Verification items for the finished model (mm, model axes). Face numbers are marked on the shaded views. A direction names the side the tool comes from. Round coordinates to 2 decimals unless told otherwise and drop trailing zeros. Order: outer loops, then holes, each group sorted by start corner. A loop starts at its lowest first (then second) coordinate and runs counter-clockwise, first axis right, second up. Notation, with made-up numbers: M 45.5,61 L 50.5,61 A25 ccw 50.5,81 Z; hole C 31.5,72 d8. An arc over 180 degrees is marked long. Use CSV: the item, a comma, the result in double quotes. Start each with the question number.
Q1. Sectioned sample at D-D (x = 16). Enter the section's corners in (y, z).
Q2. Set-up check for the marked faces 1 and 2: record each of +Z, -Z, +X, -X, +Y, -Y from which the full face is reachable in a straight line by a thin tool's end or side.
Q3. Sectioned sample at C-C (z = 18.5). Enter the section's corners in (x, y), and give its area (3 significant figures).
Q4. Mould release check, pull along Y, two halves, no side actions. Record for the marked faces 3, 4 and 5: +Y half, -Y half, draft (parallel to the pull), parting line (faces both ways), or undercut.
Q5. Gauge pin test, flat ends, axial feed: pin 1 Ø1.1 at (x, y) = (22, 124) entering from +Z; pin 2 Ø21.5 at (x, z) = (-8, -10) entering from +Y; pin 3 Ø3 at (x, y) = (21, 124.5) entering from -Z. Record the tip position at first contact, or that the pin passes through.
Q6. Sectioned sample at A-A (y = 123.5). Enter the section's corners in (x, z), and give its area (3 significant figures).
Q7. Sectioned sample at B-B (y = 91). Enter the section's corners in (x, z), and give its area (3 significant figures).
Q8. Scan lines: line 1 (Z direction, x = 20.5, y = 12); line 2 (X direction, y = 96, z = -18.5); line 3 (Y direction, x = -3.5, z = -15). Record each from-to range of solid material in increasing order.
```python
from build123d import *

# Parameters (mm, degrees)
SKETCH1_W           = 46.1
SKETCH1_H           = 51.8
SKETCH1_W_2         = 42.8
SKETCH1_H_2         = 50
BOSS_EXTRUDE1_DEPTH = 120
SKETCH2_W           = 1.65
SKETCH2_H           = 30
BOSS_EXTRUDE2_DEPTH = 12.8
BOSS_EXTRUDE5_DEPTH = 30
SKETCH6_W           = 46.1
SKETCH6_H           = 51.8
BOSS_EXTRUDE6_DEPTH = 0.8


with BuildPart() as part:
    # Sketch1 → Boss-Extrude1 (new body)
    with BuildSketch(Plane(origin=(0, 0, 0), x_dir=(1, 0, 0), z_dir=(0, 1, 0))):
        Rectangle(SKETCH1_W, SKETCH1_H)
        Rectangle(SKETCH1_W_2, SKETCH1_H_2, mode=Mode.SUBTRACT)
    extrude(amount=BOSS_EXTRUDE1_DEPTH)

    # Sketch2 → Boss-Extrude2 (add)
    with BuildSketch(Plane(origin=(0, 120, 0), x_dir=(1, 0, 0), z_dir=(0, 1, 0))):
        with Locations((22.225, 0)):
            Rectangle(SKETCH2_W, SKETCH2_H)
        with Locations((-22.225, 0)):
            Rectangle(SKETCH2_W, SKETCH2_H)
    extrude(amount=BOSS_EXTRUDE2_DEPTH)

    # Sketch5 → Boss-Extrude5 (add)
    with BuildSketch(Plane.XY.offset(15)):
        Polygon((-19.4, 130.8), (-21.4, 128), (-21.4, 132.8), align=None)
        Polygon((21.4, 128.2), (21.4, 132.8), (19.4, 130.8), align=None)
    extrude(amount=-BOSS_EXTRUDE5_DEPTH)

    # Sketch6 → Boss-Extrude6 (add)
    with BuildSketch(Plane.XZ):
        Rectangle(SKETCH6_W, SKETCH6_H)
    extrude(amount=BOSS_EXTRUDE6_DEPTH)


solid = part.part
```
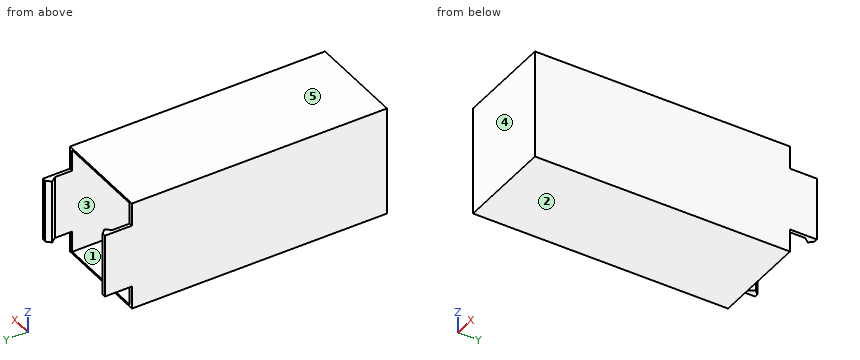
Verdict:
1,outline,"M -0.8,-25.9 L 120,-25.9 L 120,-25 L 0,-25 L 0,25 L 120,25 L 120,25.9 L -0.8,25.9 Z"
2,face 1,"+Y"
2,face 2,"-Z, +X, -X, +Y, -Y"
3,outline,"M -23.05,-0.8 L 23.05,-0.8 L 23.05,120 L 21.4,120 L 21.4,0 L -21.4,0 L -21.4,120 L -23.05,120 Z"
3,area,"433 mm²"
4,face 3,"undercut"
4,face 4,"-Y half"
4,face 5,"draft"
5,pin 1,"stops at z = 15"
5,pin 2,"stops at y = 0"
5,pin 3,"stops at z = -15"
6,outline,"M -23.05,-15 L -21.4,-15 L -21.4,15 L -23.05,15 Z; M 21.4,-15 L 23.05,-15 L 23.05,15 L 21.4,15 Z"
6,area,"99.0 mm²"
7,outline,"M -23.05,-25.9 L 23.05,-25.9 L 23.05,25.9 L -23.05,25.9 Z; hole M -21.4,-25 L 21.4,-25 L 21.4,25 L -21.4,25 Z"
7,area,"248 mm²"
8,line 1,"z = -25.9 to -25, 25 to 25.9"
8,line 2,"x = -23.05 to -21.4, 21.4 to 23.05"
8,line 3,"y = -0.8 to 0"
